from build123d import *

# Parameters (mm, degrees)
F0_W     = 425
F0_H     = 765
F0_R     = 4
F1_DEPTH = 25
F2_DEPTH = 65
F3_DEPTH = 65
F4_DEPTH = 50
F5_DEPTH = 67
F6_W     = 15.2404187247
F6_H     = 33.9140146971
F7_DEPTH = 765


with BuildPart() as f1:
    # F0 (on Front) → F1 (new body)
    with BuildSketch(Plane.XZ):
        Polygon((425, 0), (0, 0), (0, 765), (-40, 765), (-40, -40), (465, -40), (465, 765), (425, 765), align=None)
        with Locations((212.5, 382.5)):
            Rectangle(F0_W, F0_H)
        with Locations((13, 10)):
            Circle(F0_R, mode=Mode.SUBTRACT)
        with Locations((412, 10)):
            Circle(F0_R, mode=Mode.SUBTRACT)
        with Locations((13, 755)):
            Circle(F0_R, mode=Mode.SUBTRACT)
        with BuildLine():
            ThreePointArc((408, 755), (412, 759), (416, 755))
            ThreePointArc((416, 755), (414, 751.5358983849), (410, 751.5358983849))
            Line((410, 751.5358983849), (410, 90))
            Line((410, 90), (60, 90))
            Line((60, 90), (60, 755))
            Line((60, 755), (408, 755))
        make_face(mode=Mode.SUBTRACT)
    extrude(amount=F1_DEPTH)

    # F0 (on Front) → F2 (join)
    with BuildSketch(Plane.XZ):
        with BuildLine():
            Line((410, 755), (408, 755))
            ThreePointArc((408, 755), (408.5358983849, 753), (410, 751.5358983849))
            Line((410, 751.5358983849), (410, 755))
        make_face()
        with BuildLine():
            ThreePointArc((410, 751.5358983849), (414, 751.5358983849), (416, 755))
            ThreePointArc((416, 755), (412, 759), (408, 755))
            Line((408, 755), (410, 755))
            Line((410, 755), (410, 751.5358983849))
        make_face()
        with Locations((13, 755)):
            Circle(F0_R)
        with Locations((412, 10)):
            Circle(F0_R)
        with Locations((13, 10)):
            Circle(F0_R)
    extrude(amount=F2_DEPTH)

    # F0 (on Front) → F3 (join, through all)
    with BuildSketch(Plane.XZ):
        Polygon((425, 0), (0, 0), (0, 765), (-40, 765), (-40, -40), (465, -40), (465, 765), (425, 765), align=None)
    extrude(amount=F3_DEPTH)

    # F0 (on Front) → F4 (join)
    with BuildSketch(Plane.XZ):
        Polygon((425, 0), (0, 0), (0, 765), (-40, 765), (-40, -40), (465, -40), (465, 765), (425, 765), align=None)
    extrude(amount=-F4_DEPTH)

    # F0 (on Front) + F3_face (on face) → F5 (join)
    with BuildSketch(Plane.XZ):
        Polygon((425, 0), (0, 0), (0, 765), (-40, 765), (-40, -40), (465, -40), (465, 765), (425, 765), align=None)
        Polygon((-40, 765), (0, 765), (425, 765), (465, 765), (465, 805), (-40, 805), align=None)
    with BuildSketch(Plane(origin=(212.5, -65, 282.6167076167), x_dir=(1, 0, 0), z_dir=(0, -1, 0))):
        Polygon((212.5, -282.6167076167), (-212.5, -282.6167076167), (-212.5, 482.3832923833), (-252.5, 482.3832923833), (-252.5, -322.6167076167), (252.5, -322.6167076167), (252.5, 482.3832923833), (212.5, 482.3832923833), align=None)
    extrude(amount=F5_DEPTH)

    # F6 (on face) → F7 (cut, through all)
    with BuildSketch(Plane.XY.offset(765)):
        with Locations((-7.6202093624, -101.892054081)):
            Rectangle(F6_W, F6_H)
    extrude(amount=-F7_DEPTH, mode=Mode.SUBTRACT)


solid = f1.part
Source: CAD feature listing. Evaluate the final solid. Frame: model axes, mm. A direction names the side the tool comes from. Give positions to 0.01 mm unless a question says otherwise; leave off trailing zeros. Write each loop counter-clockwise with the first axis right and the second up, starting at its lowest first coordinate (ties: lowest second). Pieces come first, ordered by that corner, then holes. Notation, with made-up numbers: M 77,-26.5 L 124,-26.5 A22 cw 124,-16.5 Z; hole C -19,-10 d8. An arc over 180 degrees is marked long. Return JSON: item names as keys, results as strings. Group by question number.
1) Cut plane C-C, the plane z = 678.5. Output: boundary loops of the cut face in (x, y).
2) Cut plane B-B, the plane x = 367.5. Output: boundary loops of the cut face in (y, z).
3) Ray query, L1, parallel to X at y = 6, z = 222; L2, parallel to Z at x = 54, y = -38.5; L3, parallel to Y at x = 11.5, z = 484.5. Return the intervals inside material, ascending.
4) Cut plane A-A, the plane y = -41. Output: boundary loops of the cut face in (x, z).
5) First-contact query: pin 1 Ø25 at (x, y) = (279, 24.5) entering from +Z; pin 2 Ø4 at (x, z) = (411.5, 9.5) entering from -Y; pin 3 Ø12 at (x, z) = (224.5, 784) entering from -Y. Flat tips, straight axial feed; report the tip coordinate or a pass-through.
6) Set-up query: faces 4 (the face through (-24, -99, 765)), 5 (the face through (-8, -84.935, 388)), 6 (the face through (425, -78, 388)). Return all of +Z, -Z, +X, -X, +Y, -Y with unobstructed straight access to the full face (end or side cutting, diameter ignored); none if empty.
7) Draft query along X for faces 1 (the face through (465, -40, 377)), 2 (the face through (232, -12, 755)), 3 (the face through (216, -33, 805)). Return one class per face: released by +X, released by -X, zero draft, split by the parting line, or undercut.
Data:
{
 "1": {"outline": "M -40,-132 L 0,-132 L 0,-118.85 L -15.24,-118.85 L -15.24,-84.94 L 0,-84.94 L 0,-25 L 60,-25 L 60,0 L 0,0 L 0,50 L -40,50 Z; M 410,-25 L 425,-25 L 425,-132 L 465,-132 L 465,50 L 425,50 L 425,0 L 410,0 Z"},
 "2": {"outline": "M -132,-40 L 50,-40 L 50,0 L 0,0 L 0,90 L -25,90 L -25,0 L -132,0 Z; M -67,765 L -25,765 L -25,755 L 0,755 L 0,805 L -67,805 Z"},
 "3": {"L1": "x = -40 to 0, 425 to 465", "L2": "z = -40 to 0, 765 to 805", "L3": "y = -25 to 0"},
 "4": {"outline": "M -40,-40 L 465,-40 L 465,805 L -40,805 Z; C 13,10 d8; C 13,755 d8; C 412,10 d8; C 412,755 d8; hole M 0,0 L 425,0 L 425,765 L 0,765 Z"},
 "5": {"pin 1": "stops at z = 0", "pin 2": "stops at y = -65", "pin 3": "stops at y = -67"},
 "6": {"face 4": "+Z, +X, -X, -Y", "face 5": "+Z", "face 6": "-Y"},
 "7": {"face 1": "released by +X", "face 2": "undercut", "face 3": "zero draft"}
}
